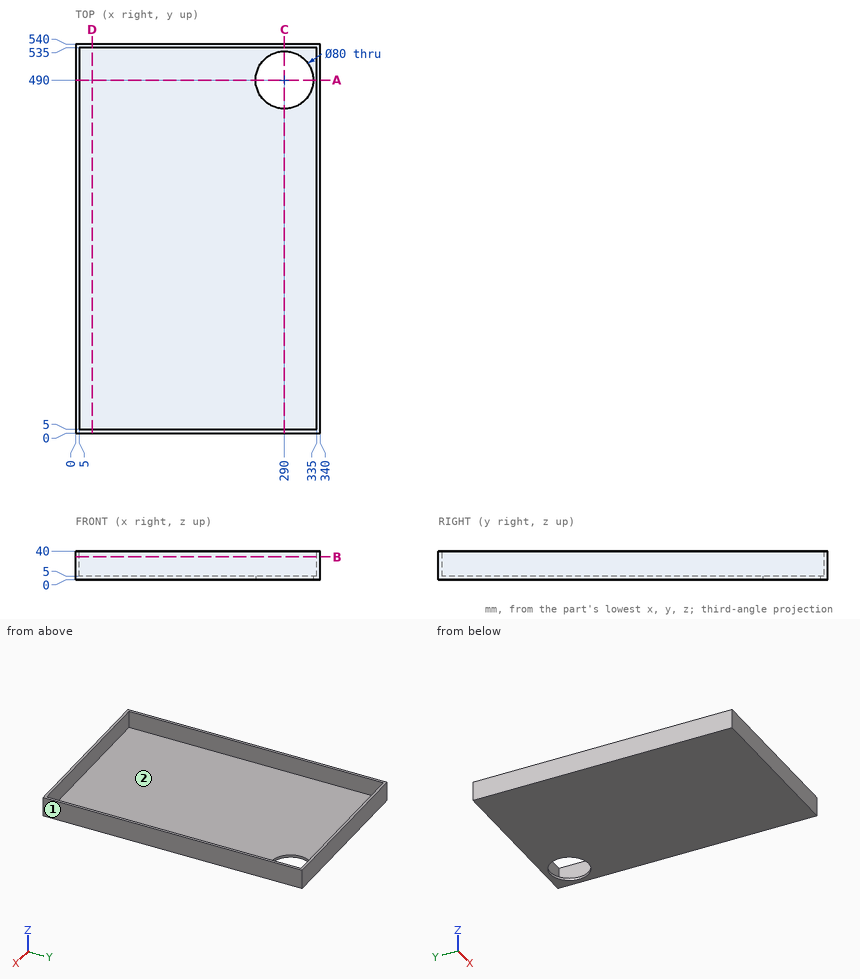
The drawing under review shows one solid part. Ordinate dimensions are in mm from its lowest x, y, z. Coordinates: 2 decimals unless noted, no trailing zeros. Order: outer loops, then holes, each group sorted by start corner. A loop starts at its lowest first (then second) coordinate and runs counter-clockwise, first axis right, second up. Notation, with made-up numbers: (-23.5, 46.5) -> (20.5, 46.5) arc R7 ccw to (20.5, 54.5) -> close; hole circle Ø2 at (-31, -25). An arc over 180 degrees is marked (long way). Return JSON: item names as keys, results as strings.
1. We need section B-B on z = 32. Write out the cut boundary in (x, y).
Answer block:
{"outline": "(0, 0) -> (340, 0) -> (340, 540) -> (0, 540) -> close; hole (5, 5) -> (335, 5) -> (335, 535) -> (5, 535) -> close"}
2. For pin 1 Ø10 at (x, y) = (36, 424.5) entering from +Z; pin 2 Ø5 at (x, z) = (41.5, 5.5) entering from -Y, all flat-tipped, find the tip position at first contact; note any pin that passes through.
Answer block:
{"pin 1": "z = 5", "pin 2": "y = 0"}
3. The part is to be moulded in two halves that separate along Y. For the marked faces 1 and 2, say which applies: +Y half, -Y half, draft (parallel to the pull), parting line (faces both ways), or undercut.
Answer block:
{"face 1": "draft", "face 2": "undercut"}
4. We need section D-D on x = 23. Write out the cut boundary in (y, z).
Answer block:
{"outline": "(0, 0) -> (540, 0) -> (540, 40) -> (535, 40) -> (535, 5) -> (5, 5) -> (5, 40) -> (0, 40) -> close"}
5. For line 1 (X direction, y = 146, z = 23); line 2 (Y direction, x = 290, z = 1); line 3 (Y direction, x = 300, z = 12.5), list the stretches that pass through material, from the lowest coordinate up. Write a range as from..to.
Answer block:
{"line 1": "0..5, 335..340", "line 2": "0..450, 530..540", "line 3": "0..5, 535..540"}
6. We need section A-A on y = 490. Write out the cut boundary in (x, z), and give its area (3 significant figures).
Answer block:
{"outline": "(0, 0) -> (250, 0) -> (250, 5) -> (5, 5) -> (5, 40) -> (0, 40) -> close; (330, 0) -> (340, 0) -> (340, 40) -> (335, 40) -> (335, 5) -> (330, 5) -> close", "area": "1,650 mm²"}
7. We need section C-C on x = 290. Write out the cut boundary in (y, z).
Answer block:
{"outline": "(0, 0) -> (450, 0) -> (450, 5) -> (5, 5) -> (5, 40) -> (0, 40) -> close; (530, 0) -> (540, 0) -> (540, 40) -> (535, 40) -> (535, 5) -> (530, 5) -> close"}
